```python
from build123d import *


with BuildPart() as part:
    # Esquisse1 → Révolution1 (revolve)
    with BuildSketch(Plane.XY):
        with BuildLine():
            Line((14.75, 0), (14.75, 30))
            Line((14.75, 30), (28.25, 35.128931493))
            Line((28.25, 35.128931493), (28.25, 46.3))
            Line((28.25, 46.3), (25.25, 46.3))
            ThreePointArc((25.25, 46.3), (12.953788056, 50.631361796), (0, 52.1))
            Line((0, 52.1), (0, 46.3))
            Line((0, 46.3), (0, -5.98683287))
            Line((0, -5.98683287), (11.203629045, -5.98683287))
            Line((11.203629045, -5.98683287), (11.203629045, 0))
            Line((11.203629045, 0), (14.75, 0))
        make_face()
    revolve(axis=Axis((0, 46.3, 0), (0, 1, 0)))


solid = part.part
```
The model under review builds one solid part; all positions refer to its coordinate system, in mm. A direction names the side the tool comes from. Round coordinates to 2 decimals unless told otherwise and drop trailing zeros. Write each loop counter-clockwise with the first axis right and the second up, starting at its lowest first coordinate (ties: lowest second). Pieces come first, ordered by that corner, then holes.
(1) We need section C-C on y = 42. Give the boundary of the cut face in (x, z), and give its area (3 significant figures).
(2) Machinability: for faces 1 (the cylindrical face through (10.686, -2.952, -3.365)), 2 (the flat face through (0, -5.987, 0)), 3 (the flat face through (-21, 46.3, 15)), which of the approach directions +Z, -Z, +X, -X, +Y, -Y give a long, thin tool a straight path to every point of the face, cutting with its end or side? Answer none if there is none.
(3) We need section A-A on x = 0. Give the boundary of the cut face in (y, z), and give its area (3 significant figures).
(4) Wall thickness on L1, parallel to Z at x = -4, y = 42.5; L2, parallel to X at y = 43.5, z = -22; L3, parallel to Z at x = 7, y = 0.5: over which ranges is each line inside the solid? List them lowest first.
(5) We need section D-D on y = 3. Give the boundary of the cut face in (x, z).
(6) We need section B-B on z = 0. Give the boundary of the cut face in (x, y).
(7) Insertion check: pin 1 (10 mm diameter, centred on y = 42, z = 7, fed in from +X); pin 2 (3 mm diameter, centred on x = 9, y = 28.5, fed in from +Z); pin 3 (6 mm diameter, centred on x = 21, z = -12, fed in from +Y); pin 4 (17 mm diameter, centred on x = 5.5, z = 2.5, fed in from +Y). Each pin has a flat end and moves straight along its axis. Give the tip position at first contact, or say it passes through.
Findings below:
1. outline: circle Ø56.5 at (0, 0)
1. area: 2,510 mm2
2. face 1: -Y
2. face 2: +Z, -Z, +X, -X, -Y
2. face 3: +Y
3. outline: (-5.99, -11.2) - (0, -11.2) - (0, -14.75) - (30, -14.75) - (35.13, -28.25) - (46.3, -28.25) - (46.3, -25.25) arc R57.86 ccw to (46.3, 25.25) - (46.3, 28.25) - (35.13, 28.25) - (30, 14.75) - (0, 14.75) - (0, 11.2) - (-5.99, 11.2) - close
3. area: 2,070 mm2
4. L1: z = -27.97 to 27.97
4. L2: x = -17.72 to 17.72
4. L3: z = -12.98 to 12.98
5. outline: circle Ø29.5 at (0, 0)
6. outline: (-28.25, 35.13) - (-14.75, 30) - (-14.75, 0) - (-11.2, 0) - (-11.2, -5.99) - (11.2, -5.99) - (11.2, 0) - (14.75, 0) - (14.75, 30) - (28.25, 35.13) - (28.25, 46.3) - (25.25, 46.3) arc R57.86 ccw to (-25.25, 46.3) - (-28.25, 46.3) - close
7. pin 1: stops at x = 28.18
7. pin 2: stops at z = 12.7
7. pin 3: stops at y = 48.08
7. pin 4: stops at y = 52.1
